Check sheet for the modelled part. Datum: model origin and axes. Units: mm. Face numbers are marked on the shaded views. A direction names the side the tool comes from. Round coordinates to 2 decimals unless told otherwise and drop trailing zeros. Loops run counter-clockwise (first coordinate to the right, second up) from the corner with the lowest first, then second, coordinate; pieces in that order, holes last. Notation, with made-up numbers: M 41,30.5 L 85,30.5 A15 cw 85,44.5 Z; hole C 72,-26 d5. An arc over 180 degrees is marked long. Write item = value, one per line. Start each with the question number.
(1) Mould release check, pull along Y, two halves, no side actions. Record for the marked faces 1, 2 and 3: pulls with the +Y half, pulls with the -Y half, needs draft (parallel to the pull), parting line crosses it, or undercut.
(2) Cross-section at A-A on x = 55. Record the boundary of the cut face in (y, z).
(3) Set-up check for the marked faces 4, 5 and 6: record each of +Z, -Z, +X, -X, +Y, -Y from which the full face is reachable in a straight line by a thin tool's end or side.
(4) Cross-section at D-D on y = -39. Record the boundary of the cut face in (x, z).
(5) Cross-section at C-C on z = 50. Record the boundary of the cut face in (x, y).
(6) Cross-section at B-B on y = -30.5. Record the boundary of the cut face in (x, z), plus the area to 3 significant figures.
(7) Go/stop test with flat-tipped pins: P1, Ø5, axis at x = 23.5, y = -2, coming from the +Z side; P2, Ø6.5, axis at y = -35.5, z = 48.5, coming from the -X side; P3, Ø12.5, axis at y = -11, z = 63, coming from the -X side; P4, Ø4, axis at x = 45, z = 88, coming from the +Y side. Record where each tip stops, or that it passes through.
(8) Scan lines: L1, parallel to X at y = 7, z = 88; L2, parallel to X at y = -30.9, z = 50; L3, parallel to Y at x = 62, z = 78. Record each from-to range of solid material in increasing order. Write a range as from..to.
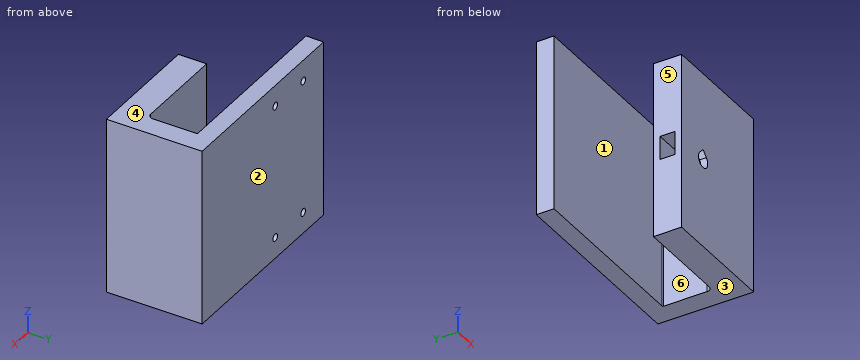
from build123d import *

# Parameters (mm, degrees)
BOSS_EXTRUDE1_DEPTH = 100
SKETCH4_R           = 4.3
CUT_EXTRUDE1_DEPTH  = 16
SKETCH5_W           = 13.3
SKETCH5_H           = 8.3
CUT_EXTRUDE2_DEPTH  = 27
SKETCH3_R           = 2.1
CUT_EXTRUDE3_DEPTH  = 8
CUT_EXTRUDE4_DEPTH  = 16
FILLET1_R           = 3
FILLET2_R           = 0.5


with BuildPart() as part:
    # Sketch1 → Boss-Extrude1 (new body)
    with BuildSketch(Plane.XY):
        Polygon((0, 0), (0, 10), (113, 10), (113, -44.3), (46, -44.3), (46, -28.3), (101, -28.3), (101, 0), align=None)
    extrude(amount=BOSS_EXTRUDE1_DEPTH)

    # Sketch4 → Cut-Extrude1 (cut)
    with BuildSketch(Plane.XZ.offset(44.3)):
        with Locations((66, 50)):
            Circle(SKETCH4_R)
    extrude(amount=-CUT_EXTRUDE1_DEPTH, mode=Mode.SUBTRACT)

    # Sketch5 → Cut-Extrude2 (cut)
    with BuildSketch(Plane.ZY.offset(-46)):
        with Locations((50, -36.3)):
            Rectangle(SKETCH5_W, SKETCH5_H)
    extrude(amount=-CUT_EXTRUDE2_DEPTH, mode=Mode.SUBTRACT)

    # Sketch3 → Cut-Extrude3 (cut)
    with BuildSketch(Plane(origin=(0, 10, 0), x_dir=(1, 0, 0), z_dir=(0, 1, 0))):
        with Locations(Location((19, -12, 0), (0, 0, 270))):
            Circle(SKETCH3_R)
        with Locations(Location((19, -88, 0), (0, 0, 270))):
            Circle(SKETCH3_R)
        with Locations(Location((45, -12, 0), (0, 0, 270))):
            Circle(SKETCH3_R)
        with Locations(Location((45, -88, 0), (0, 0, 270))):
            Circle(SKETCH3_R)
    extrude(amount=-CUT_EXTRUDE3_DEPTH, mode=Mode.SUBTRACT)

    # Sketch6 → Cut-Extrude4 (cut)
    with BuildSketch(Plane.XZ.offset(44.3)):
        Polygon((66, 56.08), (62.96, 53.04), (66, 50), (69.04, 53.04), align=None)
    extrude(amount=-CUT_EXTRUDE4_DEPTH, mode=Mode.SUBTRACT)

    # Fillet1
    fillet1_edges = [part.edges().sort_by_distance(p)[0] for p in [
        (101, -28.3, 50),
    ]]
    fillet(fillet1_edges, radius=FILLET1_R)

    # Fillet2
    fillet2_edges = [part.edges().sort_by_distance(p)[0] for p in [
        (101, 0, 50),
    ]]
    fillet(fillet2_edges, radius=FILLET2_R)


solid = part.part
Result:
q1.face_1 = undercut
q1.face_2 = pulls with the +Y half
q1.face_3 = needs draft
q2.outline = M -44.3,0 L -28.3,0 L -28.3,100 L -44.3,100 Z; M 0,0 L 10,0 L 10,100 L 0,100 Z; hole M -40.45,43.35 L -32.15,43.35 L -32.15,56.65 L -40.45,56.65 Z
q3.face_4 = +Z, +X, -X, +Y, -Y
q3.face_5 = +Z, -Z, -X, -Y
q3.face_6 = +Z, -Z, -X
q4.outline = M 46,0 L 113,0 L 113,100 L 46,100 L 46,56.65 L 73,56.65 L 73,43.35 L 46,43.35 Z
q5.outline = M 0,0 L 100.5,0 A0.5 cw 101,-0.5 L 101,-25.3 A3 cw 98,-28.3 L 70.3,-28.3 L 70.3,-32.15 L 73,-32.15 L 73,-40.45 L 70.3,-40.45 L 70.3,-44.3 L 113,-44.3 L 113,10 L 0,10 Z; M 46,-44.3 L 61.7,-44.3 L 61.7,-40.45 L 46,-40.45 Z; M 46,-32.15 L 61.7,-32.15 L 61.7,-28.3 L 46,-28.3 Z
q6.outline = M 46,0 L 113,0 L 113,100 L 46,100 Z; hole M 63.02,53.1 A4.3 ccw long 68.98,53.1 L 66,56.08 Z
q6.area = 6,640 mm^2
q7.P1 = 100
q7.P2 = 73
q7.P3 = 101
q7.P4 = 2
q8.L1 = 0..16.9, 21.1..42.9, 47.1..113
q8.L2 = 46..61.7, 70.3..113
q8.L3 = -44.3..-28.3, 0..10
